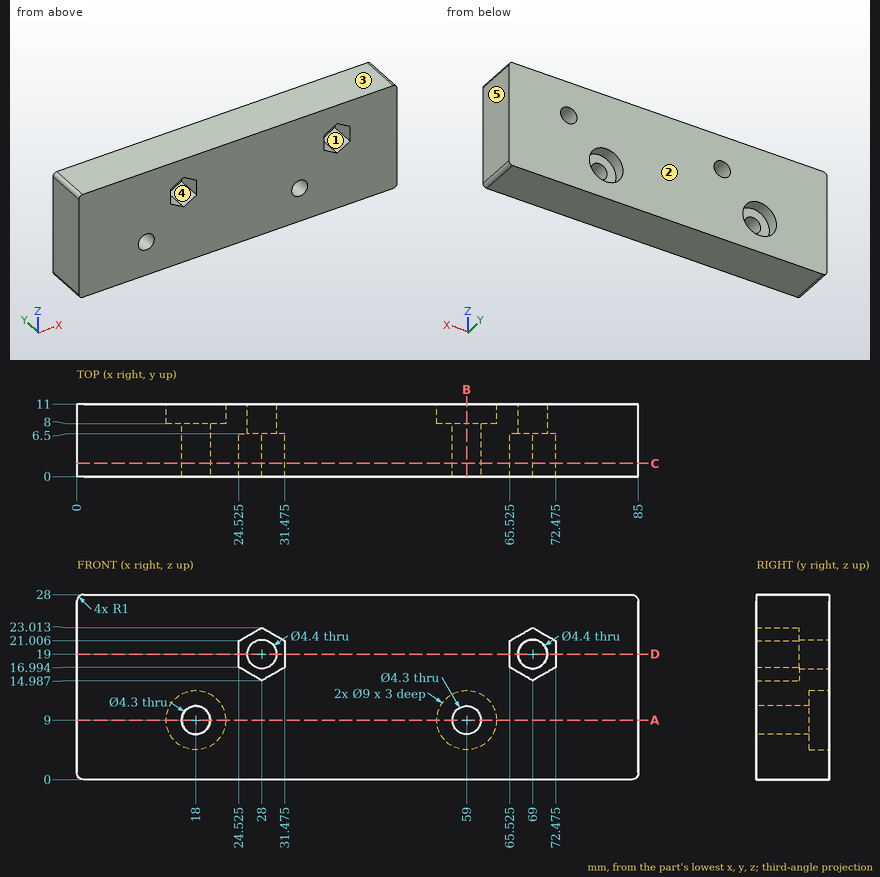
For this review, use the dimensioned drawing (mm, ordinates from the lowest corner) and the shaded views. A direction names the side the tool comes from. Round coordinates to 2 decimals unless told otherwise and drop trailing zeros. Order: outer loops, then holes, each group sorted by start corner. A loop starts at its lowest first (then second) coordinate and runs counter-clockwise, first axis right, second up. Notation, with made-up numbers: (-33, -33.75) -> (-13, -33.75) arc R3 ccw to (-13, -29.75) -> close; hole circle Ø1 at (66.5, 10). An arc over 180 degrees is marked (long way). One line per item, written item: value. Start each with the question number.
Q1. Machinability: for the marked faces 1 and 2, which of the approach directions +Z, -Z, +X, -X, +Y, -Y give a long, thin tool a straight path to every point of the face, cutting with its end or side? Answer none if there is none.
Q2. Clearance check with flat-ended pins moving along their axes: pin 1 Ø4.5 at (x, z) = (18.5, 9) entering from +Y; pin 2 Ø2.5 at (x, z) = (28, 19) entering from +Y. State where each tip first meets the part, or that it passes through.
Q3. Mouldability with a two-part tool opening along Z and no side actions: class the marked faces 3, 4 and 5 as released by +Z, released by -Z, zero draft, split by the parting line, or undercut.
Q4. Take a section at A-A (z = 9). Write out the cut boundary in (x, y), and give its area (3 significant figures).
Q5. Take a section at C-C (y = 2). Count the separate pieces of the cut face and the enclosed holes in it, and give its area (3 significant figures).
Q6. Take a section at B-B (x = 59). Write out the cut boundary in (y, z).
Q7. Take a section at D-D (z = 19). Write out the cut boundary in (x, y) (1 decimal).
Q8. Wall thickness on line 1 (X direction, y = 9.35, z = 19); line 2 (Z direction, x = 28, y = 7.9); line 3 (Z direction, x = 59, y = 4): over which ranges is each line inside the solid? List them lowest first.
Reported:
1. face 1: -Y
1. face 2: +Z, -Z, +X, -X, +Y
2. pin 1: stops at y = 8
2. pin 2: passes through
3. face 3: released by +Z
3. face 4: undercut
3. face 5: zero draft
4. outline: (0, 0) -> (15.85, 0) -> (15.85, 8) -> (13.5, 8) -> (13.5, 11) -> (0, 11) -> close; (20.15, 0) -> (56.85, 0) -> (56.85, 8) -> (54.5, 8) -> (54.5, 11) -> (22.5, 11) -> (22.5, 8) -> (20.15, 8) -> close; (61.15, 0) -> (85, 0) -> (85, 11) -> (63.5, 11) -> (63.5, 8) -> (61.15, 8) -> close
4. area: 812 mm2
5. separate pieces: 1
5. enclosed holes: 4
5. area: 2,270 mm2
6. outline: (0, 0) -> (11, 0) -> (11, 4.5) -> (8, 4.5) -> (8, 6.85) -> (0, 6.85) -> close; (0, 11.15) -> (8, 11.15) -> (8, 13.5) -> (11, 13.5) -> (11, 28) -> (0, 28) -> close
7. outline: (0, 0) -> (24.5, 0) -> (24.5, 6.5) -> (25.8, 6.5) -> (25.8, 11) -> (0, 11) -> close; (30.2, 6.5) -> (31.5, 6.5) -> (31.5, 0) -> (65.5, 0) -> (65.5, 6.5) -> (66.8, 6.5) -> (66.8, 11) -> (30.2, 11) -> close; (71.2, 6.5) -> (72.5, 6.5) -> (72.5, 0) -> (85, 0) -> (85, 11) -> (71.2, 11) -> close
8. line 1: x = 0 to 25.8, 30.2 to 66.8, 71.2 to 85
8. line 2: z = 0 to 16.8, 21.2 to 28
8. line 3: z = 0 to 6.85, 11.15 to 28
